from build123d import *

# Parameters (mm, degrees)
SKETCH_1_R          = 4.1
SKETCH_1_R_2        = 2.5
EXTRUDE_1_DEPTH     = 20
SKETCH_2_W          = 20
SKETCH_2_H          = 140
CUT_EXTRUDE_1_DEPTH = 169.819430161
FILLET_1_R          = 10
SKETCH_3_W          = 20
SKETCH_3_H          = 20
EXTRUDE_2_DEPTH     = 10
SKETCH_4_W          = 20
SKETCH_4_H          = 20
EXTRUDE_3_DEPTH     = 10
SKETCH_5_R          = 2.1
CUT_EXTRUDE_2_DEPTH = 169.819430161


with BuildPart() as part:
    # ｽｹｯﾁ1 → ﾎﾞｽ - 押し出し1 (new body)
    with BuildSketch(Plane(origin=(0, 0, 0), x_dir=(1, 0, 0), z_dir=(0, 1, 0))):
        with BuildLine():
            Line((-50, 0), (50, 0))
            Line((50, 0), (50, 150))
            ThreePointArc((50, 150), (47.071067812, 157.071067812), (40, 160))
            Line((40, 160), (-40, 160))
            ThreePointArc((-40, 160), (-47.071067812, 157.071067812), (-50, 150))
            Line((-50, 150), (-50, 0))
        make_face()
        with Locations(Location((-30, 20, 0), (0, 0, 270))):
            Circle(SKETCH_1_R, mode=Mode.SUBTRACT)
        with Locations(Location((30, 20, 0), (0, 0, 270))):
            Circle(SKETCH_1_R, mode=Mode.SUBTRACT)
        with Locations(Location((-42, 32, 0), (0, 0, 270))):
            Circle(SKETCH_1_R_2, mode=Mode.SUBTRACT)
        with Locations(Location((-18, 32, 0), (0, 0, 270))):
            Circle(SKETCH_1_R_2, mode=Mode.SUBTRACT)
        with Locations(Location((-18, 8, 0), (0, 0, 270))):
            Circle(SKETCH_1_R_2, mode=Mode.SUBTRACT)
        with Locations(Location((-42, 8, 0), (0, 0, 270))):
            Circle(SKETCH_1_R_2, mode=Mode.SUBTRACT)
        with Locations(Location((18, 32, 0), (0, 0, 90))):
            Circle(SKETCH_1_R_2, mode=Mode.SUBTRACT)
        with Locations(Location((18, 8, 0), (0, 0, 90))):
            Circle(SKETCH_1_R_2, mode=Mode.SUBTRACT)
        with Locations(Location((42, 8, 0), (0, 0, 90))):
            Circle(SKETCH_1_R_2, mode=Mode.SUBTRACT)
        with Locations(Location((42, 32, 0), (0, 0, 90))):
            Circle(SKETCH_1_R_2, mode=Mode.SUBTRACT)
    extrude(amount=EXTRUDE_1_DEPTH)

    # ｽｹｯﾁ2 → ｶｯﾄ - 押し出し1 (cut, through all)
    with BuildSketch(Plane(origin=(0, 20, 0), x_dir=(1, 0, 0), z_dir=(0, 1, 0))):
        with Locations((0, 70)):
            Rectangle(SKETCH_2_W, SKETCH_2_H)
    extrude(amount=-CUT_EXTRUDE_1_DEPTH, mode=Mode.SUBTRACT)

    # ﾌｨﾚｯﾄ1
    fillet_1_edges = [part.edges().sort_by_distance(p)[0] for p in [
        (-10, 10, -140),
        (10, 10, -140),
    ]]
    fillet(fillet_1_edges, radius=FILLET_1_R - 0.0001)  # a hair under: the kernel refuses the full size

    # ｽｹｯﾁ3 → ﾎﾞｽ - 押し出し2 (add)
    with BuildSketch(Plane.XY):
        with Locations((30, 10)):
            Rectangle(SKETCH_3_W, SKETCH_3_H)
    extrude(amount=EXTRUDE_2_DEPTH)

    # ｽｹｯﾁ4 → ﾎﾞｽ - 押し出し3 (add)
    with BuildSketch(Plane.XY):
        with Locations((-30, 10)):
            Rectangle(SKETCH_4_W, SKETCH_4_H)
    extrude(amount=EXTRUDE_3_DEPTH)

    # ｽｹｯﾁ5 → ｶｯﾄ - 押し出し2 (cut, through all)
    with BuildSketch(Plane(origin=(0, 20, 0), x_dir=(1, 0, 0), z_dir=(0, 1, 0))):
        with Locations(Location((20, 102, 0), (0, 0, 270))):
            Circle(SKETCH_5_R)
        with Locations(Location((40, 102, 0), (0, 0, 270))):
            Circle(SKETCH_5_R)
        with Locations(Location((20, 78, 0), (0, 0, 270))):
            Circle(SKETCH_5_R)
        with Locations(Location((40, 78, 0), (0, 0, 270))):
            Circle(SKETCH_5_R)
    extrude(amount=-CUT_EXTRUDE_2_DEPTH, mode=Mode.SUBTRACT)


solid = part.part
Could you check a few things on this model? Use its own coordinates, in mm. A direction names the side the tool comes from. Give positions to 0.01 mm unless a question says otherwise; leave off trailing zeros. Order: outer loops, then holes, each group sorted by start corner. A loop starts at its lowest first (then second) coordinate and runs counter-clockwise, first axis right, second up.
Item 1: For faces 1 (the face through (7.15, 9.86, -136.99)), 2 (the face through (40, 10, 5)), 3 (the face through (-45, 10, 0)), 4 (the face through (47.15, 9.86, -156.99)), which set-ups out of +Z, -Z, +X, -X, +Y, -Y let a thin tool reach every point of the face, with its end or its side?
Item 2: If we section it at D-D, the plane x = 30: Write out the boundary of the cut face in (y, z).
Item 3: If we section it at B-B, the plane y = 13: Count the separate pieces of the cut face and the enclosed holes in it, plus the area to 3 significant figures.
Item 4: If we section it at A-A, the plane z = -59: Write out the boundary of the cut face in (x, y), plus the area to 3 significant figures.
Item 5: I'm going to push flat-ended pins straight in: pin 1 (4.5 mm diameter, centred on x = -18, z = -32, fed in from -Y); pin 2 (3 mm diameter, centred on y = 12.5, z = 6, fed in from -X); pin 3 (3 mm diameter, centred on y = 10, z = 7.5, fed in from +X); pin 4 (5 mm diameter, centred on x = -2, y = 15, fed in from +Z). Where does each tip first touch, or does it pass through?
Item 6: If we section it at C-C, the plane z = -78: Write out the boundary of the cut face in (x, y).
Item 7: If we mould it in two halves opening along X, with no side actions, what happens to faces 5 (the face through (30, 10, 10)), 6 (the face through (20.09, 10.14, -104.1)), 7 (the face through (-40, 10, 5))? For each: pulls with the +X half, pulls with the -X half, needs draft (parallel to the pull), parting line crosses it, or undercut.
Item 8: I need wall thicknesses on line 1 (X direction, y = 14.5, z = -8); line 2 (X direction, y = 11.75, z = -126); line 3 (X direction, y = 14.75, z = -102). Which ranges of each line are inside material? Lowest first, please.
Values:
1. face 1: +Z, +Y, -Y
1. face 2: +Z, +X, +Y, -Y
1. face 3: +Z, -X, +Y, -Y
1. face 4: -Z, +X, +Y, -Y
2. outline: (0, -160) - (20, -160) - (20, -24.1) - (0, -24.1) - close; (0, -15.9) - (20, -15.9) - (20, 10) - (0, 10) - close
3. separate pieces: 1
3. enclosed holes: 14
3. area: 13,300 mm2
4. outline: (-50, 0) - (-10, 0) - (-10, 20) - (-50, 20) - close; (10, 0) - (50, 0) - (50, 20) - (10, 20) - close
4. area: 1,600 mm2
5. pin 1: passes through
5. pin 2: stops at x = -40
5. pin 3: stops at x = 40
5. pin 4: stops at z = -138.93
6. outline: (-50, 0) - (-10, 0) - (-10, 20) - (-50, 20) - close; (10, 0) - (17.9, 0) - (17.9, 20) - (10, 20) - close; (22.1, 0) - (37.9, 0) - (37.9, 20) - (22.1, 20) - close; (42.1, 0) - (50, 0) - (50, 20) - (42.1, 20) - close
7. face 5: needs draft
7. face 6: undercut
7. face 7: pulls with the -X half
8. line 1: x = -50 to -44.5, -39.5 to -20.5, -15.5 to -10, 10 to 15.5, 20.5 to 39.5, 44.5 to 50
8. line 2: x = -50 to -10, 10 to 50
8. line 3: x = -50 to -10, 10 to 17.9, 22.1 to 37.9, 42.1 to 50
